from build123d import *

# Parameters (mm, degrees)
FILLET1_R = 0.79375


with BuildPart() as part:
    # Sketch1 → Revolve1 (revolve)
    with BuildSketch(Plane.XY):
        Polygon((-15.24, 21.59), (-15.24, 0), (0, 0), (0, 2.54), (-12.7, 2.54), (-12.7, 21.59), align=None)
    revolve(axis=Axis((0, 0, 0), (0, 1, 0)))

    # Fillet1
    fillet1_edges = [part.edges().sort_by_distance(p)[0] for p in [
        (12.7, 21.59, 0),
        (12.7, 2.54, 0),
        (15.24, 0, 0),
        (15.24, 21.59, 0),
    ]]
    fillet(fillet1_edges, radius=FILLET1_R)

    # Sketch4 → CSK for #10 Flat Head Machine Screw (100)1 (revolve, cut)
    with BuildSketch(Plane(origin=(0, 2.54, 0), x_dir=(0, 0, 1), z_dir=(1, 0, 0))):
        Polygon((0, 0), (0, 2.54), (2.5527, 2.54), (2.5527, 1.960808018), (4.8895, 0), align=None)
    revolve(axis=Axis((0, 8.89, 0), (0, -1, 0)), mode=Mode.SUBTRACT)


solid = part.part
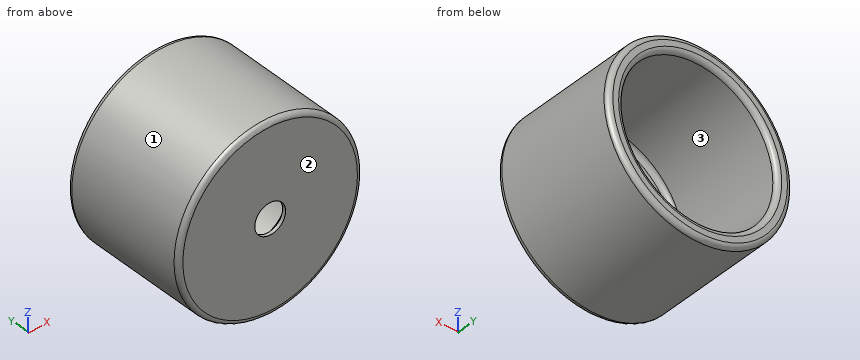
Could you check a few things on this model? Use its own coordinates, in mm. Face numbers are marked on the shaded views. Give positions to 0.01 mm unless a question says otherwise; leave off trailing zeros. Write each loop counter-clockwise with the first axis right and the second up, starting at its lowest first coordinate (ties: lowest second). Pieces come first, ordered by that corner, then holes. Notation, with made-up numbers: (87, -13.5) - (98, -13.5) arc R17 ccw to (98, 1.5) - close; hole circle Ø3 at (26.5, 25.25). An arc over 180 degrees is marked (long way). Use CSV: the item, a comma, the result in double quotes. Start each with the question number.
Item 1: If I drill on line 1 along Z through (x, y) = (0, 10); line 2 along X through (y, z) = (5.25, -7); line 3 along X through (y, z) = (8.25, -10.5), over which ranges is the centre line in solid material (lowest first)?
Item 2: I want a section at A-A, the plane z = 0. Please give me the cut outline in (x, y), then the cut area to 3 significant figures.
Item 3: If we mould it in two halves opening along Z, with no side actions, what happens to the marked faces 1, 2 and 3? For each: pulls with the +Z half, pulls with the -Z half, needs draft (parallel to the pull), parting line crosses it, or undercut.
Item 4: I'm going to push flat-ended pins straight in: pin 1 (3 mm diameter, centred on x = -2.5, z = -8, fed in from -Y); pin 2 (1 mm diameter, centred on x = -5.5, z = -7.5, fed in from +Y); pin 3 (8 mm diameter, centred on x = 9.5, y = 15, fed in from +Z); pin 4 (4.5 mm diameter, centred on x = 0, z = 0, fed in from +Y). Where does each tip first touch, or does it pass through?
Item 5: I want a section at C-C, the plane y = 10.5. Please give me the cut outline in (x, z).
Item 6: I want a section at B-B, the plane x = 0. Please give me the cut outline in (y, z).
Findings:
1,line 1,"z = -15.24 to -12.7, 12.7 to 15.24"
1,line 2,"x = -13.54 to -10.6, 10.6 to 13.54"
1,line 3,"x = -11.05 to -7.14, 7.14 to 11.05"
2,outline,"(-15.24, 0.79) arc R0.79 ccw to (-14.45, 0) - (-2.55, 0) - (-2.55, 0.58) - (-4.89, 2.54) - (-11.91, 2.54) arc R0.79 cw to (-12.7, 3.33) - (-12.7, 20.8) arc R0.79 ccw to (-13.49, 21.59) - (-14.45, 21.59) arc R0.79 ccw to (-15.24, 20.8) - close; (2.55, 0) - (14.45, 0) arc R0.79 ccw to (15.24, 0.79) - (15.24, 20.8) arc R0.79 ccw to (14.45, 21.59) - (13.49, 21.59) arc R0.79 ccw to (12.7, 20.8) - (12.7, 3.33) arc R0.79 cw to (11.91, 2.54) - (4.89, 2.54) - (2.55, 0.58) - close"
2,area,"156 mm2"
3,face 1,"parting line crosses it"
3,face 2,"needs draft"
3,face 3,"undercut"
4,pin 1,"stops at y = 0"
4,pin 2,"stops at y = 2.54"
4,pin 3,"stops at z = 14.21"
4,pin 4,"passes through"
5,outline,"circle Ø30.48 at (0, 0); hole circle Ø25.4 at (0, 0)"
6,outline,"(0, -14.45) arc R0.79 ccw to (0.79, -15.24) - (20.8, -15.24) arc R0.79 ccw to (21.59, -14.45) - (21.59, -13.49) arc R0.79 ccw to (20.8, -12.7) - (3.33, -12.7) arc R0.79 cw to (2.54, -11.91) - (2.54, -4.89) - (0.58, -2.55) - (0, -2.55) - close; (0, 2.55) - (0.58, 2.55) - (2.54, 4.89) - (2.54, 11.91) arc R0.79 cw to (3.33, 12.7) - (20.8, 12.7) arc R0.79 ccw to (21.59, 13.49) - (21.59, 14.45) arc R0.79 ccw to (20.8, 15.24) - (0.79, 15.24) arc R0.79 ccw to (0, 14.45) - close"
